Autodesk Inventor part; units mm, degrees
ref_plane "Work Plane1" through (0, 26, 0) normal (0, 1, 0) x (1, 0, 0)
ref_plane "YZ Plane" through (0, 0, 0) normal (1, 0, 0) x (0, 1, 0)
ref_plane "XZ Plane" through (0, 0, 0) normal (0, 1, 0) x (-1, 0, 0)
sketch "Sketch1" plane through (0, 0, 0) normal (0, 0, 1) x (1, 0, 0)
  line L0 (0, 0) -> (0, 8)
  line L1 (-3.5, 0) -> (-3.5, 16)
  line L2 (-3.5, 16) -> (-6, 16)
  line L3 (-6, 16) -> (-6, 10.1213)
  line L4 (-6, 10.1213) -> (-15.3787, 19.5)
  line L5 (-3.5, 0) -> (-6, 0)
  line L6 (-6, 0) -> (-6, 5.8787)
  line L7 (-6, 5.8787) -> (-19.3813, 19.26)
  line L8 (-19.3813, 19.26) -> (-19.3813, 31.5)
  line L9 (-19.3813, 31.5) -> (-18, 31.5)
  line L10 (-6, 10.1213) -> (-6, 5.8787)
  line L11 (-6, 8) -> (0, 8)
  line L12 (-15.3787, 19.5) -> (-15.3787, 26)
  line L13 (-15.3787, 26) -> (-18, 26)
  line L14 (-18, 26) -> (-18, 31.5)
  dimension "d0" = 7
  dimension "d1" = 12
  dimension "d2" = 45
  dimension "d3" = 16
  dimension "d5" = 12.24
  dimension "d6" = 3
  dimension "d7" = 31.5
  dimension "d8" = 8
  dimension "d28" = 36
  dimension "d29" = 12
  dimension "d30" = 6.5
revolve "Revolution1" add sketch "Sketch1" angle 360 about axis through (0, 0, 0) along (0, 1, 0)
ref_plane "Work Plane1" through (0, 26, 0) normal (0, 1, 0) x (1, 0, 0)
sketch "Sketch2" plane through (0, 26, 0) normal (0, 1, 0) x (1, 0, 0)
  circle A0 centre (-16, 0) radius 2.75
  line L0 (0, 0) -> (0, 15.3787)
  circle A1 centre (0, 0) radius 15.3787
  circle A2 centre (16, 0) radius 2.75
  point P0 (15.1544, 2.6168)
  point P1 (15.1544, -2.6168)
  point P2 (-15.1544, 2.6168)
  point P3 (-15.1544, -2.6168)
  point P4 (-15.1544, 2.6168)
  point P5 (-15.1544, -2.6168)
  dimension "d11" = 32
  dimension "d12" = 5.5
  dimension "d35" = 5.2335
extrude "Extrusion1" add sketch "Sketch2" against normal up to surface contours A0 A1 | A2 A1 picked at (-14.6525, 0) picked at (14.7143, -0.6004)
sketch "Sketch3" plane through (0, 26, 0) normal (0, 1, 0) x (1, 0, 0)
  arc A0 (-15.1544, -2.6168) -> (-15.1544, 2.6168) centre (-16, 0) ccw
  arc A1 (15.1544, 2.6168) -> (15.1544, -2.6168) centre (16, 0) ccw
  point P0 (0, 0)
  point P1 (-17.8887, -1.9989)
  point P2 (-17.8887, 1.9989)
  point P3 (17.8887, 1.9989)
  point P4 (17.8887, -1.9989)
sketch "Sketch4" plane through (0, 0, 0) normal (0, 0, 1) x (1, 0, 0)
  circle A0 centre (-18, 26.2) radius 0.2
  line L0 (0, 25.76) -> (0, 31.5)
  line L1 (18, 26) -> (-18, 26)
  line L2 (-18, 31.5) -> (-18, 26)
  point P0 (0, 0)
  point P1 (-15.1544, 26)
  dimension "d15" = 0.4
revolve "Revolution2" cut sketch "Sketch4" angle 360 about axis through (0, 25.76, 0) along (0, 1, 0)
hole "Hole1" at (-16, 26, 0) at (16, 26, 0) direction (0, -1, 0) diameter 2.013 depth 7 tip angle 118
sketch "Sketch7" plane through (0, 31.5, 0) normal (0, 1, 0) x (1, 0, 0)
  line L0 (31.4446, -31.0263) -> (0, -31.0263)
  line L1 (0, -31.0263) -> (0, 28.9425)
  line L2 (0, 28.9425) -> (31.4446, 28.9425)
  line L3 (31.4446, 28.9425) -> (31.4446, -31.0263)
  point P0 (0, 0)
properties part number "18102021-002-08" material "Stainless Steel"
Source: CAD feature listing. Evaluate the final solid. Frame: model axes, mm. A direction names the side the tool comes from. Round coordinates to 2 decimals unless told otherwise and drop trailing zeros. Write each loop counter-clockwise with the first axis right and the second up, starting at its lowest first coordinate (ties: lowest second). Pieces come first, ordered by that corner, then holes. Notation, with made-up numbers: M 38.25,-1 L 54.25,-1 A31 cw 54.25,33 Z; hole C 65.25,-6 d1. An arc over 180 degrees is marked long. One line per item, written item: value. Start each with the question number.
Item 1: Section query A-A (x = 0). Return the cut outline in (y, z).
Item 2: Pin query (flat end, axial travel): pin 1 (10 mm diameter, centred on x = 11, y = 17.5, fed in from -Z); pin 2 (4 mm diameter, centred on x = 8.5, z = 11, fed in from -Y); pin 3 (12 mm diameter, centred on y = 20.5, z = 7.5, fed in from -X); pin 4 (4 mm diameter, centred on x = 0, z = 0, fed in from +Y). Return the tip coordinate at first contact, or that it passes through.
Item 3: Ray query, L1, parallel to X at y = 30, z = 0.5; L2, parallel to Z at x = -3, y = 6.5; L3, parallel to Z at x = 0, y = 9. Return the intervals inside material, ascending. Write a range as from..to.
Item 4: Mould query, pull axis X, two halves, no side actions, for faces 1 (the flat face through (-3, 0, -3)), 2 (the conical face through (-16.11, 18.5, -0.14)), 3 (the cylindrical face through (4.2, 25.47, -18.92)). Classes: pulls with the +X half, pulls with the -X half, needs draft (parallel to the pull), parting line crosses it, or undercut.
Item 5: Set-up query: faces 4 (the cylindrical face through (0.301, 22.796, -15.376)), 5 (the cylindrical face through (6, 3, 0)), 6 (the cylindrical face through (-3.233, 8.112, -1.341)). Return all of +Z, -Z, +X, -X, +Y, -Y with unobstructed straight access to the full face (end or side cutting, diameter ignored); none if empty.
Result set:
1. outline: M 0,-6 L 5.88,-6 L 19.26,-19.38 L 31.5,-19.38 L 31.5,-18 L 26.4,-18 A0.2 cw 26,-18 L 26,-15.38 L 19.5,-15.38 L 10.12,-6 L 16,-6 L 16,-3.5 L 0,-3.5 Z; M 0,3.5 L 16,3.5 L 16,6 L 10.12,6 L 19.5,15.38 L 26,15.38 L 26,18 A0.2 cw 26.4,18 L 31.5,18 L 31.5,19.38 L 19.26,19.38 L 5.88,6 L 0,6 Z
2. pin 1: stops at z = -18.32
2. pin 2: stops at y = 11.78
2. pin 3: stops at x = -19.32
2. pin 4: passes through
3. L1: x = -19.37..-17.99, 17.99..19.37
3. L2: z = -5.9..-1.8, 1.8..5.9
3. L3: z = -9.12..-3.5, 3.5..9.12
4. face 1: needs draft
4. face 2: undercut
4. face 3: parting line crosses it
5. face 4: +Y
5. face 5: -Y
5. face 6: +Y, -Y
